CAD build for the part. Positions are in the model's coordinates, mm. A direction names the side the tool comes from. Coordinates: 2 decimals unless noted, no trailing zeros. Order: outer loops, then holes, each group sorted by start corner. A loop starts at its lowest first (then second) coordinate and runs counter-clockwise, first axis right, second up.
from build123d import *

# Parameters (mm, degrees)
F0_R             = 50.5
F1_DEPTH         = 3
F2_R             = 50.5
F2_R_2           = 49.4440908639
F3_DEPTH         = 50
F4_R             = 12.5
F5_DEPTH         = 50
F6_SIZE          = 1
F9_R             = 4.6632476683
F10_DEPTH        = 53.001
F10_COPIES_COUNT = 10
F10_COPIES_ANGLE = 141.4287
F11_R            = 4.0917082841
F11_R_2          = 3.0111553801
F11_R_3          = 2.1424193095
F12_DEPTH        = 53.001


# Not quite as in the source:
# - a pattern or mirror of a feature is missing from the dataset's text; its kind, count and spacing are read off the source's solid


with BuildPart() as f1:
    # F0 (on Front) → F1 (new body)
    with BuildSketch(Plane.XZ):
        Circle(F0_R)
    extrude(amount=F1_DEPTH)

    # F2 (on face) → F3 (join)
    with BuildSketch(Plane.XZ.offset(3)):
        Circle(F2_R)
        Circle(F2_R_2, mode=Mode.SUBTRACT)
    extrude(amount=F3_DEPTH)

    # F4 (on face) → F5 (join)
    with BuildSketch(Plane.XZ.offset(3)):
        Circle(F4_R)
    extrude(amount=F5_DEPTH)

    # F6
    f6_edges = [f1.edges().sort_by_distance(p)[0] for p in [
        (-12.5, -53, 0),
    ]]
    chamfer(f6_edges, length=F6_SIZE)

    # F9 (on face) → F10 (cut, through all)
    with BuildSketch(Plane(origin=(0, 0, 0), x_dir=(-1, 0, 0), z_dir=(0, 1, 0))):
        with Locations((0, -44.030174613)):
            Circle(F9_R)
    f10 = extrude(amount=-F10_DEPTH, mode=Mode.SUBTRACT)

    # F10_copies: F10 ×10 about axis
    f10_copies_axis = Axis((0, 0, 0), (0, 1, 0))
    for i in range(1, F10_COPIES_COUNT):
        add(f10.rotate(f10_copies_axis, i * F10_COPIES_ANGLE / (F10_COPIES_COUNT - 1)), mode=Mode.SUBTRACT)

    # F10_copies1: F10 across plane
    add(f10.mirror(Plane(origin=(0, 0, 0), x_dir=(0.9801724878, 0, 0.1981461432), z_dir=(-0.1981461432, 0, 0.9801724878))), mode=Mode.SUBTRACT)

    # F10_copies2: F10 across plane
    add(f10.mirror(Plane(origin=(0, 0, 0), x_dir=(0.9980579158, 0, 0.0622928302), z_dir=(-0.0622928302, 0, 0.9980579158))), mode=Mode.SUBTRACT)

    # F10_copies3: F10 across plane
    add(f10.mirror(Plane(origin=(0, 0, 0), x_dir=(0.9972037972, 0, -0.0747300936), z_dir=(0.0747300936, 0, 0.9972037972))), mode=Mode.SUBTRACT)

    # F10_copies4: F10 across plane
    add(f10.mirror(Plane(origin=(0, 0, 0), x_dir=(0.9776261689, 0, -0.2103498843), z_dir=(0.2103498843, 0, 0.9776261689))), mode=Mode.SUBTRACT)

    # F10_copies5: F10 across plane
    add(f10.mirror(Plane(origin=(0, 0, 0), x_dir=(0.9396926208, 0, -0.3420201433), z_dir=(0.3420201433, 0, 0.9396926208))), mode=Mode.SUBTRACT)

    # F11 (on face) → F12 (cut, through all)
    with BuildSketch(Plane(origin=(0, 0, 0), x_dir=(-1, 0, 0), z_dir=(0, 1, 0))):
        with Locations((-9.1548590747, 32.8874919017)):
            Circle(F11_R)
        with Locations((-6.3979976493, 22.98387055)):
            Circle(F11_R_2)
        with Locations((-4.3693644676, 15.6963026268)):
            Circle(F11_R_3)
        with Locations((-10.4730058489, 12.4812423457)):
            Circle(F11_R_3)
        with Locations((-15.3354720805, 18.2761039461)):
            Circle(F11_R_2)
        with Locations((-21.9434412824, 26.1511749822)):
            Circle(F11_R)
        with Locations((5.2749524196, 33.7279327151)):
            Circle(F11_R)
        with Locations((3.686472168, 23.5712240313)):
            Circle(F11_R_2)
        with Locations((2.5175908752, 16.0974220976)):
            Circle(F11_R_3)
        with Locations((18.7591014711, 28.5218281367)):
            Circle(F11_R)
        with Locations((13.1100529385, 19.9328671126)):
            Circle(F11_R_2)
        with Locations((8.9532073342, 13.6126904187)):
            Circle(F11_R_3)
        with Locations((28.8802291505, 18.2024979735)):
            Circle(F11_R)
        with Locations((20.1833405306, 12.7210630218)):
            Circle(F11_R_2)
        with Locations((13.7837454444, 8.6875556704)):
            Circle(F11_R_3)
        with Locations((33.8238792195, 4.6199310394)):
            Circle(F11_R)
        with Locations((25.7207452383, -22.4464213773)):
            Circle(F11_R)
        with Locations((17.9752922715, -15.6869865537)):
            Circle(F11_R_2)
        with Locations((32.7037831717, -9.7908699573)):
            Circle(F11_R)
        with Locations((22.855483208, -6.8424824959)):
            Circle(F11_R_2)
        with Locations((14.1266433863, -31.0779104011)):
            Circle(F11_R)
        with BuildLine():
            ThreePointArc((0, -30.0462261622), (-2.8932746743, -37.0312091207), (4.0917082841, -34.1379344463))
            ThreePointArc((4.0917082841, -34.1379344463), (2.8932746743, -31.244659772), (0, -30.0462261622))
        make_face()
        with BuildLine():
            ThreePointArc((0, -20.8466039317), (-3.0111553801, -23.8577593118), (0, -26.8689146919))
            Line((0, -26.8689146919), (0, -20.8466039317))
        make_face()
        with BuildLine():
            Line((0, -20.8466039317), (0, -26.8689146919))
            ThreePointArc((0, -26.8689146919), (2.1292083885, -25.9869677003), (3.0111553801, -23.8577593118))
            ThreePointArc((3.0111553801, -23.8577593118), (2.1292083885, -21.7285509233), (0, -20.8466039317))
        make_face()
        with Locations((9.8725966659, -21.7192199319)):
            Circle(F11_R_2)
        with BuildLine():
            ThreePointArc((0, -14.1506854285), (-2.1424193095, -16.293104738), (0, -18.4355240475))
            Line((0, -18.4355240475), (0, -14.1506854285))
        make_face()
        with BuildLine():
            Line((0, -14.1506854285), (0, -18.4355240475))
            ThreePointArc((0, -18.4355240475), (1.5149192219, -17.8080239599), (2.1424193095, -16.293104738))
            ThreePointArc((2.1424193095, -16.293104738), (1.5149192219, -14.7781855161), (0, -14.1506854285))
        make_face()
        with Locations((6.7422614761, -14.8326387468)):
            Circle(F11_R_3)
        with Locations((12.2758099722, -10.7130645256)):
            Circle(F11_R_3)
        with Locations((15.6086234621, -4.6729151098)):
            Circle(F11_R_3)
        with Locations((23.6382775495, 3.2287015768)):
            Circle(F11_R_2)
        with Locations((16.1432147465, 2.2049670412)):
            Circle(F11_R_3)
    extrude(amount=-F12_DEPTH, mode=Mode.SUBTRACT)


solid = f1.part
1) Drill centre lines: probe 1 along X at (y, z) = (-41, -5); probe 2 along Z at (x, y) = (6, -40); probe 3 along Z at (x, y) = (4, -41.5). Where is each one in solid material? Low to high.
2) Two-plate mould, pull along X, no slides. Class faces 1 (the flat face through (37.2, -53, -33.4)), 2 (the cylindrical face through (-15.763, -1.479, 7.867)), 3 (the flat face through (10, -3, -10)): released by +X, released by -X, zero draft, split by the parting line, or undercut.
3) Slice it at A-A (x = 28.5). List the corners of the cut face in (y, z).
4) Which spindle directions (+Z, -Z, +X, -X, +Y, -Y) get a long thin tool onto all of the face, cutting with end or side? Do faces 4 (the cylindrical face through (-10.72, -27.65, -48.27)), 5 (the cylindrical face through (-36.822, -1.479, 16.07)). Say none if no direction does.
5) Pin check, flat tips, straight feed: P1, Ø4, axis at y = -22, z = -9.5, coming from the +X side; P2, Ø10, axis at y = -24.5, z = -29, coming from the +X side; P3, Ø1.5, axis at y = -14.5, z = 33.5, coming from the -X side. Stop position of each tip, or through.
6) Slice it at B-B (y = -12.5). List the corners of the cut face in (x, z).
Worked out:
1. probe 1: x = -50.25 to -49.19, -11.46 to 11.46, 49.19 to 50.25
1. probe 2: z = -50.14 to -49.08, -10.97 to 10.97, 49.08 to 50.14
1. probe 3: z = -50.34 to -49.28, -11.84 to 11.84, 49.28 to 50.34
2. face 1: zero draft
2. face 2: undercut
2. face 3: undercut
3. outline: (-53, -41.69) - (0, -41.69) - (0, 29.07) - (-3, 29.07) - (-3, -40.4) - (-53, -40.4) - close; (-53, 40.4) - (-3, 40.4) - (-3, 38.39) - (0, 38.39) - (0, 41.69) - (-53, 41.69) - close
4. face 4: -Y
4. face 5: +Y, -Y
5. P1: stops at x = 49.94
5. P2: stops at x = 44.43
5. P3: stops at x = -38.44
6. outline: circle Ø101 at (0, 0); circle Ø25 at (0, 0); hole circle Ø98.89 at (0, 0)
